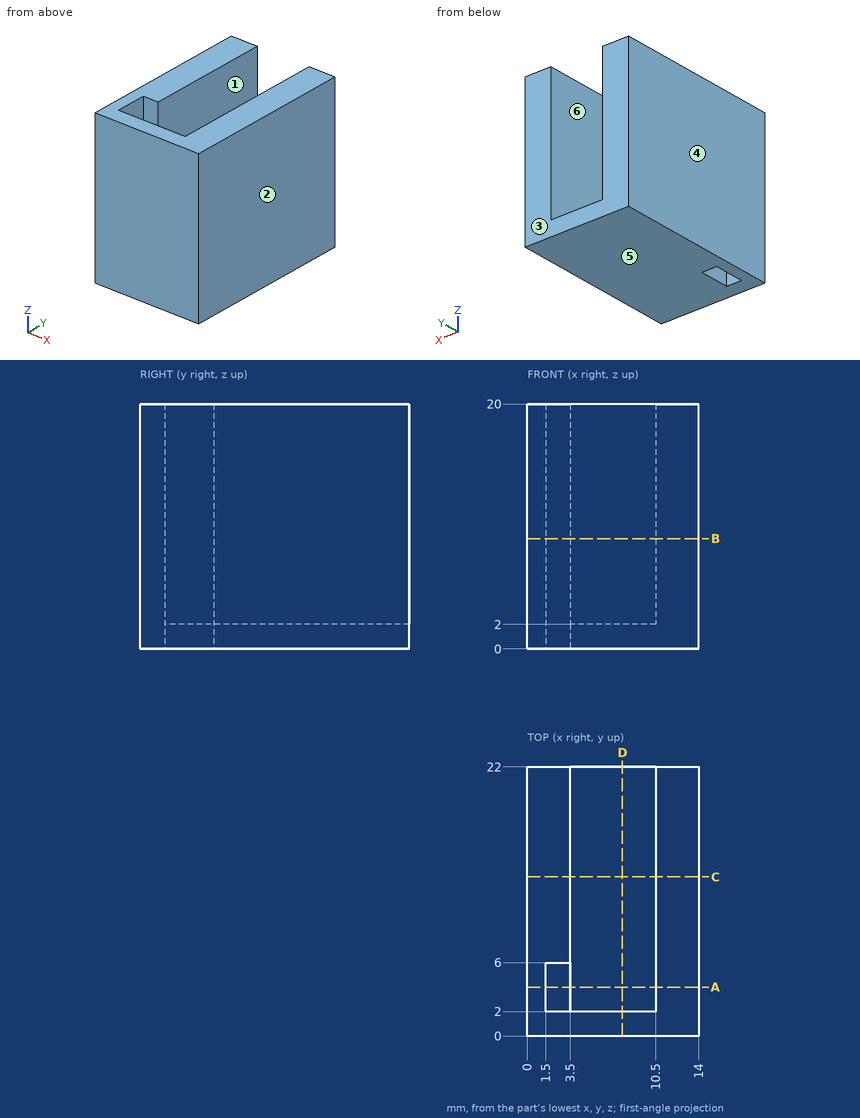
For this review, use the dimensioned drawing (mm, ordinates from the lowest corner) and the shaded views. A direction names the side the tool comes from. Round coordinates to 2 decimals unless told otherwise and drop trailing zeros. Write each loop counter-clockwise with the first axis right and the second up, starting at its lowest first coordinate (ties: lowest second). Pieces come first, ordered by that corner, then holes. Notation, with made-up numbers: (-14.5, 0.5) - (13.5, 0.5) arc R27 cw to (13.5, 34.5) - close; hole circle Ø7 at (87.25, 17). An arc over 180 degrees is marked (long way). Answer as a JSON object with one key per item and string values.
1. We need section D-D on x = 7.75. Give the boundary of the cut face in (y, z).
Response values:
{"outline": "(0, 0) - (22, 0) - (22, 2) - (2, 2) - (2, 20) - (0, 20) - close"}
2. To check wall thickness, follow line 1 along X through (y, z) = (6.75, 17.5); line 2 along Y through (x, z) = (2, 6.25); line 3 along X through (y, z) = (4.5, 9.5). State the ranges of each line that lie inside material, in increasing order.
Response values:
{"line 1": "x = 0 to 3.5, 10.5 to 14", "line 2": "y = 0 to 2, 6 to 22", "line 3": "x = 0 to 1.5, 10.5 to 14"}
3. We need section C-C on y = 13. Give the boundary of the cut face in (x, z).
Response values:
{"outline": "(0, 0) - (14, 0) - (14, 20) - (10.5, 20) - (10.5, 2) - (3.5, 2) - (3.5, 20) - (0, 20) - close"}
4. We need section A-A on y = 4. Give the boundary of the cut face in (x, z).
Response values:
{"outline": "(0, 0) - (1.5, 0) - (1.5, 20) - (0, 20) - close; (3.5, 0) - (14, 0) - (14, 20) - (10.5, 20) - (10.5, 2) - (3.5, 2) - close"}
5. Draft analysis for pull direction X (two halves, no side actions). For the marked faces 1, 2, 3 and 4, state which applies: +X half, -X half, draft (parallel to the pull), parting line (faces both ways), or undercut.
Response values:
{"face 1": "undercut", "face 2": "+X half", "face 3": "draft", "face 4": "-X half"}
6. Tool access review of the marked faces 5 and 6: name each direction out of +Z, -Z, +X, -X, +Y, -Y from which nothing blocks a thin tool from reaching the whole face with its end or side.
Response values:
{"face 5": "-Z, +X, -X, +Y, -Y", "face 6": "+Z, +Y"}
7. We need section B-B on z = 9. Give the boundary of the cut face in (x, y).
Response values:
{"outline": "(0, 0) - (14, 0) - (14, 22) - (10.5, 22) - (10.5, 2) - (1.5, 2) - (1.5, 6) - (3.5, 6) - (3.5, 22) - (0, 22) - close"}
